The drawing under review shows one solid part. Ordinate dimensions are in mm from its lowest x, y, z. A direction names the side the tool comes from. Round coordinates to 2 decimals unless told otherwise and drop trailing zeros. Write each loop counter-clockwise with the first axis right and the second up, starting at its lowest first coordinate (ties: lowest second). Pieces come first, ordered by that corner, then holes.
Item 1: Add section D-D (z = 48.5). Give the boundary of the cut face in (x, y).
Item 2: Draft analysis for pull direction Y (two halves, no side actions). For the marked faces 1, 2 and 3, state which applies: +Y half, -Y half, draft (parallel to the pull), parting line (faces both ways), or undercut.
Item 3: Add section C-C (y = 22). Give the boundary of the cut face in (x, z) (1 decimal), plus the area to 3 significant figures.
Item 4: Clearance check with flat-ended pins moving along their axes: pin 1 Ø9.5 at (x, y) = (30.24, 23.87) entering from +Z; pin 2 Ø12 at (y, z) = (19.01, 28.82) entering from +X; pin 3 Ø12 at (x, z) = (23.5, 27) entering from +Y. State where each tip first meets the part, or that it passes through.
Item 5: To check wall thickness, follow L1, parallel to X at y = 37, z = 17; L2, parallel to Y at x = 29, z = 6. State the ranges of each line that lie inside material, in increasing order.
Item 6: Machinability: for the marked faces 4, 5, 6 and 7, which of the approach directions +Z, -Z, +X, -X, +Y, -Y give a long, thin tool a straight path to every point of the face, cutting with its end or side? Answer none if there is none.
Item 7: Add section B-B (x = 15.5). Give the boundary of the cut face in (y, z), plus the area to 3 significant figures.
Item 8: Add section A-A (y = 33.5). Give the boundary of the cut face in (x, z).
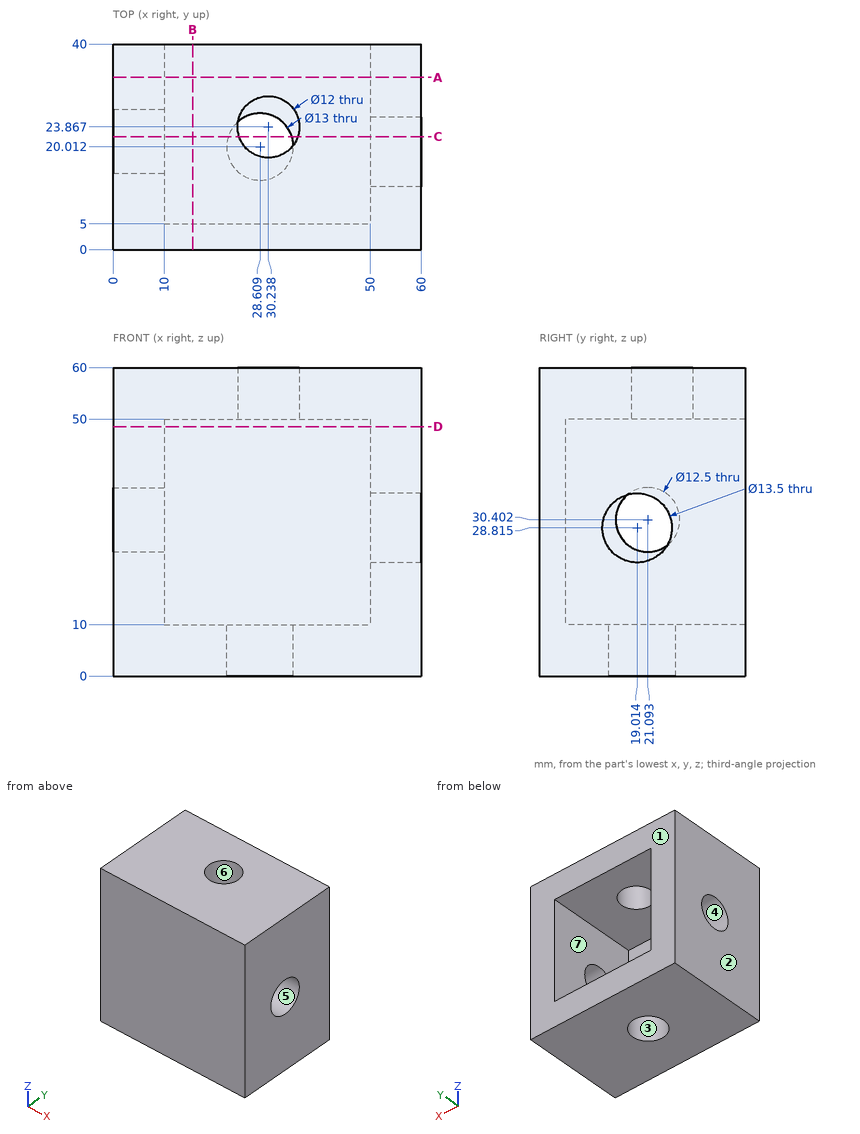
Numbers:
1. outline: (0, 0) - (60, 0) - (60, 40) - (50, 40) - (50, 5) - (10, 5) - (10, 40) - (0, 40) - close
2. face 1: +Y half
2. face 2: draft
2. face 3: undercut
3. outline: (0, 0) - (22.4, 0) - (22.4, 10) - (10, 10) - (10, 24.2) - (0, 24.2) - close; (0, 36.6) - (10, 36.6) - (10, 50) - (24.5, 50) - (24.5, 60) - (0, 60) - close; (34.8, 0) - (60, 0) - (60, 22.8) - (50, 22.8) - (50, 10) - (34.8, 10) - close; (35.9, 50) - (50, 50) - (50, 34.9) - (60, 34.9) - (60, 60) - (35.9, 60) - close
3. area: 1,520 mm2
4. pin 1: stops at z = 10
4. pin 2: stops at x = 10
4. pin 3: stops at y = 5
5. L1: x = 0 to 10, 50 to 60
5. L2: y = 0 to 13.52, 26.5 to 40
6. face 4: -X
6. face 5: +X
6. face 6: +Z
6. face 7: +Y
7. outline: (0, 0) - (40, 0) - (40, 10) - (5, 10) - (5, 50) - (40, 50) - (40, 60) - (0, 60) - close
7. area: 1,000 mm2
8. outline: (0, 0) - (60, 0) - (60, 60) - (0, 60) - close; hole (10, 10) - (50, 10) - (50, 50) - (10, 50) - close
